The figure shows three views and two pictorial views of one solid part (mm, origin at its lowest corner). Answer the questions. A direction names the side the tool comes from. Coordinates: 2 decimals unless noted, no trailing zeros. Loops run counter-clockwise (first coordinate to the right, second up) from the corner with the lowest first, then second, coordinate; pieces in that order, holes last. Notation, with made-up numbers: (67.25, 5.25) - (86.25, 5.25) arc R10 ccw to (86.25, 21.25) - close; hole circle Ø11 at (83, 69.25). An arc over 180 degrees is marked (long way). Return JSON: item names as keys, results as strings. Group by question number.
1. Section B-B (x = 80) is taken. Write down the section's boundary in (y, z), and give its area (3 significant figures).
2. Section A-A (y = 12.5) is taken. Write down the section's boundary in (x, z).
3. Which of the six approach directions +Z, -Z, +X, -X, +Y, -Y give full straight-line access (tool end or side, diameter ignored) to the marked faces 1, 2, 3 and 4?
4. Each of these flat-tipped pins is pushed along its axis until it touches: P1, Ø3, axis at x = 73, y = 6.5, coming from the +Z side; P2, Ø1.5, axis at x = 28, z = 36, coming from the +Y side; P3, Ø1, axis at y = 5.5, z = 17.5, coming from the +X side; P4, Ø1.5, axis at x = 47, z = 55.5, coming from the +Y side. Where does it stop, or does it pass through?
5. Section D-D (x = 44) is taken. Write down the section's boundary in (y, z), and give its area (4 significant figures).
6. Section C-C (z = 67.5) is taken. Write down the section's boundary in (x, y).
7. Find the intervals of material crossed by line 1 along X through (y, z) = (3, 57.5); line 2 along Z through (x, y) = (28.5, 5), in increasing order.
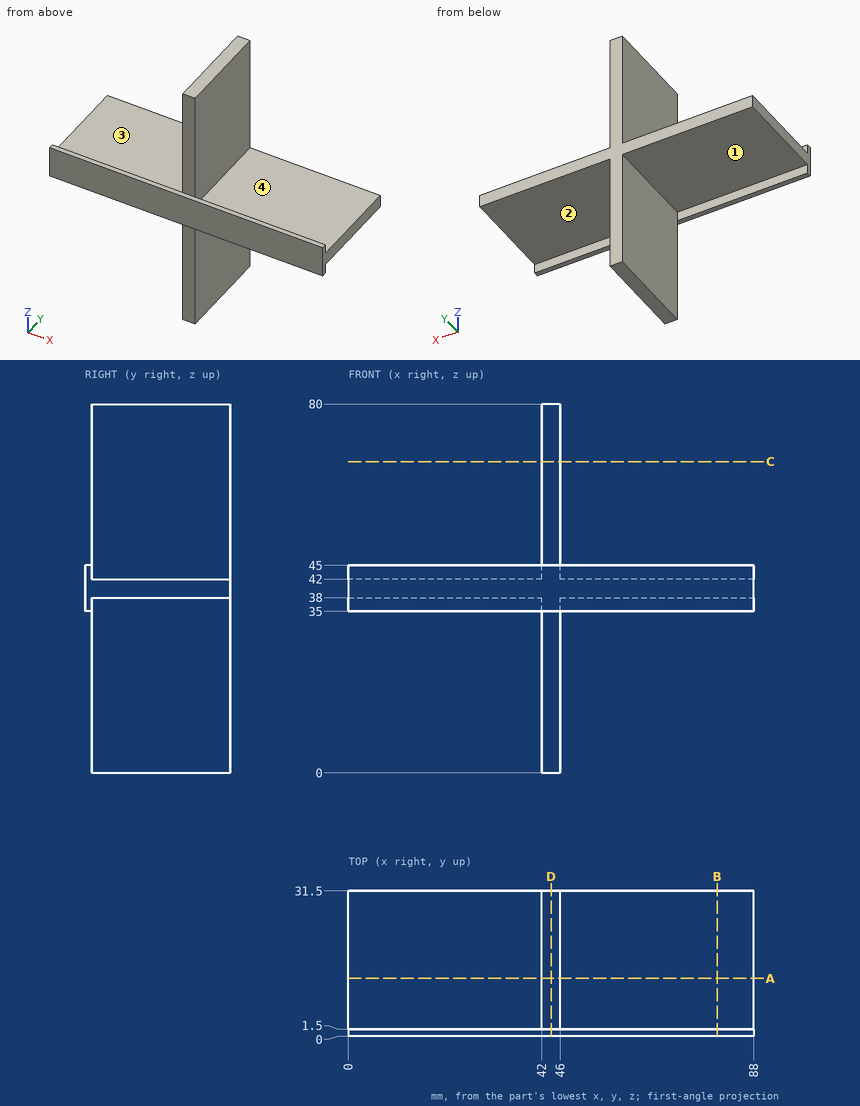
The answers:
{
 "1": {"outline": "(0, 35) - (1.5, 35) - (1.5, 38) - (31.5, 38) - (31.5, 42) - (1.5, 42) - (1.5, 45) - (0, 45) - close", "area": "135 mm2"},
 "2": {"outline": "(0, 38) - (42, 38) - (42, 0) - (46, 0) - (46, 38) - (88, 38) - (88, 42) - (46, 42) - (46, 80) - (42, 80) - (42, 42) - (0, 42) - close"},
 "3": {"face 1": "-Z, -X, +Y", "face 2": "-Z, +X, +Y", "face 3": "+Z, -X, +Y", "face 4": "+Z, +X, +Y"},
 "4": {"P1": "stops at z = 42", "P2": "stops at y = 1.5", "P3": "stops at x = 46", "P4": "passes through"},
 "5": {"outline": "(0, 35) - (1.5, 35) - (1.5, 0) - (31.5, 0) - (31.5, 80) - (1.5, 80) - (1.5, 45) - (0, 45) - close", "area": "2,415 mm2"},
 "6": {"outline": "(42, 1.5) - (46, 1.5) - (46, 31.5) - (42, 31.5) - close"},
 "7": {"line 1": "x = 42 to 46", "line 2": "z = 38 to 42"}
}
